Verification items for the finished model (mm, model axes). Face numbers are marked on the shaded views. A direction names the side the tool comes from. Round coordinates to 2 decimals unless told otherwise and drop trailing zeros. Loops run counter-clockwise (first coordinate to the right, second up) from the corner with the lowest first, then second, coordinate; pieces in that order, holes last. Notation, with made-up numbers: (-2.75, 7.25) - (24.25, 7.25) arc R17 cw to (24.25, 31.25) - close; hole circle Ø1 at (-18, 87). An arc over 180 degrees is marked (long way). Use CSV: the item, a comma, the result in double quotes.
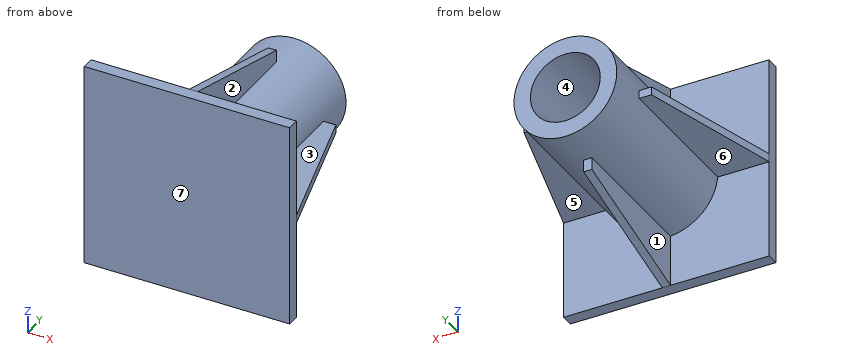
Autodesk Inventor part; units mm, degrees
ref_plane "YZ Plane" through (0, 0, 0) normal (1, 0, 0) x (0, 1, 0)
ref_plane "XZ Plane" through (0, 0, 0) normal (0, 1, 0) x (-1, 0, 0)
ref_plane "XY Plane" through (0, 0, 0) normal (0, 0, 1) x (1, 0, 0)
sketch "Sketch1" plane through (0, 0, 0) normal (0, 1, 0) x (-1, 0, 0)
  circle A0 centre (0, 0) radius 12.5
  circle A1 centre (0, 0) radius 8.5
  dimension "d0" = 25
  dimension "d1" = 4
extrude "Extrusion1" add sketch "Sketch1" against normal blind 45
sketch "Sketch2" plane through (0, -45, 0) normal (0, -1, 0) x (1, 0, 0)
  line L0 (-25, -25) -> (25, -25)
  line L1 (25, -25) -> (25, 25)
  line L2 (25, 25) -> (-25, 25)
  line L3 (-25, 25) -> (-25, -25)
  line L4 (-25, -25) -> (25, 25) construction
  line L5 (25, -25) -> (-25, 25) construction
  point P0 (0, 0)
  dimension "d4" = 50
  dimension "d5" = 50
extrude "Extrusion2" add sketch "Sketch2" along normal blind 3
sketch "Sketch3" plane through (0, 0, 0) normal (1, 0, 0) x (0, 1, 0)
  line L0 (0, -12.5) -> (-45, -12.5) construction
  line L1 (-45, 25) -> (-45, -25) construction
  line L2 (-10, -12.5) -> (-45, -12.5)
  line L3 (-45, -12.5) -> (-45, -15.5)
  line L4 (-45, -15.5) -> (-10, -15.5)
  line L5 (-10, -15.5) -> (-10, -12.5)
  line L6 (-10, -15.5) -> (-45, -25)
  line L7 (-45, -25) -> (-45, -15.5)
  point P0 (0, 0)
  dimension "d8" = 3
  dimension "d9" = 10
extrude "Extrusion3" add sketch "Sketch3" along normal mid plane 2
pattern_circular "Circular Pattern1" count 4 over 360 about axis through (0, -10, 0) along (0, 1, 0) of "Extrusion3"
properties part number "pin_sleeve"
1) Mould release check, pull along X, two halves, no side actions. Record for the marked faces 1, 2, 3 and 4: +X half, -X half, draft (parallel to the pull), parting line (faces both ways), or undercut.
Returned:
face 1,"-X half"
face 2,"+X half"
face 3,"draft"
face 4,"undercut"
2) Cross-section at B-B, the plane x = -10. Record the cut outline in (y, z), then the cut area to 3 significant figures.
Returned:
outline,"(-48, -25) - (-45, -25) - (-45, -7.5) - (0, -7.5) - (0, 7.5) - (-45, 7.5) - (-45, 25) - (-48, 25) - close"
area,"825 mm²"
3) Access from +Z, -Z, +X, -X, +Y, -Y to the whole of each face (thin tool, end or side, straight path). Record for the marked faces 5, 6 and 7.
Returned:
face 5,"-Z, +X, +Y"
face 6,"-Z, -X, +Y"
face 7,"+Z, -Z, +X, -X, -Y"
4) Gauge pin test, flat ends, axial feed: pin 1 Ø12 at (y, z) = (-38, 16.5) entering from +X; pin 2 Ø1 at (x, y) = (-6.5, -21.5) entering from -Z; pin 3 Ø2 at (x, z) = (0, -14) entering from +Y; pin 4 Ø12.5 at (x, z) = (-10.5, 7.5) entering from +Y. Record the tip position at first contact, or that the pin passes through.
Returned:
pin 1,"stops at x = 6.78"
pin 2,"stops at z = -10.97"
pin 3,"stops at y = -10"
pin 4,"stops at y = 0"
5) Cross-section at C-C, the plane z = 13.5. Record the cut outline in (x, y), then the cut area to 3 significant figures.
Returned:
outline,"(-25, -48) - (25, -48) - (25, -45) - (1, -45) - (1, -10) - (-1, -10) - (-1, -45) - (-25, -45) - close"
area,"220 mm²"
6) Thickness scan on probe 1 along Y at (x, z) = (17, 17); probe 2 along X at (y, z) = (-27.5, 4); probe 3 along Z at (x, y) = (-7, -25.5). Record the ranges inside material, lowest first. Write a range as [from, to].
Returned:
probe 1,"y = [-48, -45]"
probe 2,"x = [-11.84, -7.5], [7.5, 11.84]"
probe 3,"z = [-10.36, -4.82], [4.82, 10.36]"
